Geometry: final body of the model. Coordinates: model frame, mm. A direction names the side the tool comes from. Round coordinates to 2 decimals unless told otherwise and drop trailing zeros. Order: outer loops, then holes, each group sorted by start corner. A loop starts at its lowest first (then second) coordinate and runs counter-clockwise, first axis right, second up. Notation, with made-up numbers: (69.5, -1.5) -> (115.5, -1.5) arc R13 ccw to (115.5, 7.5) -> close; hole circle Ø1 at (13, 31.5). An arc over 180 degrees is marked (long way). Put each result on its own line as item: value.
```python
from build123d import *

# Parameters (mm, degrees)
F1_DEPTH = 15.875
F3_DEPTH = 25.4
F5_DEPTH = 25.4


with BuildPart() as f1:
    # F0 (on Front) → F1 (new body)
    with BuildSketch(Plane.XZ):
        Polygon((-45.72, 0), (0, 0), (0, 12.7), (-36.195, 12.7), (-36.195, 63.5), (-45.72, 63.5), align=None)
    extrude(amount=F1_DEPTH)

    # F2 (on face) → F3 (cut)
    with BuildSketch(Plane.XY.offset(12.7)):
        with BuildLine():
            Line((-10.795, -5.3975), (-31.115, -5.3975))
            ThreePointArc((-31.115, -5.3975), (-33.655, -7.9375), (-31.115, -10.4775))
            Line((-31.115, -10.4775), (-10.795, -10.4775))
            ThreePointArc((-10.795, -10.4775), (-8.255, -7.9375), (-10.795, -5.3975))
        make_face()
    extrude(amount=-F3_DEPTH, mode=Mode.SUBTRACT)

    # F4 (on face) → F5 (cut)
    with BuildSketch(Plane(origin=(0, 0, 0), x_dir=(-1, 0, 0), z_dir=(0, 1, 0))):
        with BuildLine():
            ThreePointArc((24.13, 12.7), (25.4, 11.43), (26.67, 12.7))
            Line((26.67, 12.7), (24.13, 12.7))
        make_face()
        with BuildLine():
            Line((30.48, 12.7), (27.94, 12.7))
            ThreePointArc((27.94, 12.7), (29.21, 11.43), (30.48, 12.7))
        make_face()
        with BuildLine():
            ThreePointArc((20.32, 12.7), (21.59, 11.43), (22.86, 12.7))
            Line((22.86, 12.7), (20.32, 12.7))
        make_face()
        with BuildLine():
            Line((34.29, 12.7), (31.75, 12.7))
            ThreePointArc((31.75, 12.7), (33.02, 11.43), (34.29, 12.7))
        make_face()
        with BuildLine():
            ThreePointArc((16.51, 12.7), (17.78, 11.43), (19.05, 12.7))
            Line((19.05, 12.7), (16.51, 12.7))
        make_face()
        with BuildLine():
            ThreePointArc((12.7, 12.7), (13.97, 11.43), (15.24, 12.7))
            Line((15.24, 12.7), (12.7, 12.7))
        make_face()
        with BuildLine():
            ThreePointArc((8.89, 12.7), (10.16, 11.43), (11.43, 12.7))
            Line((11.43, 12.7), (8.89, 12.7))
        make_face()
        with BuildLine():
            ThreePointArc((5.08, 12.7), (6.35, 11.43), (7.62, 12.7))
            Line((7.62, 12.7), (5.08, 12.7))
        make_face()
        with BuildLine():
            Line((3.81, 12.7), (1.27, 12.7))
            ThreePointArc((1.27, 12.7), (2.54, 11.43), (3.81, 12.7))
        make_face()
        with BuildLine():
            ThreePointArc((3.81, 12.7), (2.54, 13.97), (1.27, 12.7))
            Line((1.27, 12.7), (3.81, 12.7))
        make_face()
    extrude(amount=-F5_DEPTH, mode=Mode.SUBTRACT)


solid = f1.part
```
1. Cut plane D-D on x = -6.35. Return loops of the section in (y, z) (3 decimals), and give its area (3 significant figures).
Ans:
outline: (-15.875, 0) -> (0, 0) -> (0, 11.43) -> (-15.875, 11.43) -> close
area: 181 mm²
2. Cut plane B-B on y = -12.75. Return loops of the section in (x, z) (3 decimals), and give its area (3 significant figures).
Ans:
outline: (-45.72, 0) -> (0, 0) -> (0, 12.7) -> (-1.27, 12.7) arc R1.27 cw to (-3.81, 12.7) -> (-5.08, 12.7) arc R1.27 cw to (-7.62, 12.7) -> (-8.89, 12.7) arc R1.27 cw to (-11.43, 12.7) -> (-12.7, 12.7) arc R1.27 cw to (-15.24, 12.7) -> (-16.51, 12.7) arc R1.27 cw to (-19.05, 12.7) -> (-20.32, 12.7) arc R1.27 cw to (-22.86, 12.7) -> (-24.13, 12.7) arc R1.27 cw to (-26.67, 12.7) -> (-27.94, 12.7) arc R1.27 cw to (-30.48, 12.7) -> (-31.75, 12.7) arc R1.27 cw to (-34.29, 12.7) -> (-36.195, 12.7) -> (-36.195, 63.5) -> (-45.72, 63.5) -> close
area: 1,040 mm²
3. Set-up query: faces 1 (the face through (-23, -11, 0)), 2 (the face through (-33.654, -7.882, 6.439)), 3 (the face through (-35, -8, 12.7)). Return all of +Z, -Z, +X, -X, +Y, -Y with unobstructed straight access to the full face (end or side cutting, diameter ignored); none if empty.
Ans:
face 1: -Z, +X, -X, +Y, -Y
face 2: +Z, -Z
face 3: +Z, +X, +Y, -Y
4. Material intervals for probe 1 along X at (y, z) = (-15, 14.5) (3 decimals); probe 2 along Z at (x, y) = (-10, -12.25); probe 3 along Z at (x, y) = (-4, -2), sorted ascending.
Ans:
probe 1: -45.72 to -36.195
probe 2: 0 to 11.44
probe 3: 0 to 12.7
5. Cut plane C-C on z = 39.5. Return loops of the section in (x, y) (3 decimals), and give its area (3 significant figures).
Ans:
outline: (-45.72, -15.875) -> (-36.195, -15.875) -> (-36.195, 0) -> (-45.72, 0) -> close
area: 151 mm²
6. Contact query for flat-ended pins moving along their axis: P1, Ø1, axis at x = -12, y = -13.5, coming from the +Z side; P2, Ø1, axis at y = -12, z = 55.5, coming from the +X side (3 decimals). Output: stop coordinate, or through.
Ans:
P1: z = 12.7
P2: x = -36.195
7. Draft query along X for faces 4 (the face through (-38, 0, 18)), 5 (the face through (-13.94, -13.14, 11.43)), 6 (the face through (0, -8, 6)). Return one class per face: +X half, -X half, draft (parallel to the pull), parting line (faces both ways), or undercut.
Ans:
face 4: draft
face 5: undercut
face 6: +X half
8. Cut plane A-A on x = -29.21. Return loops of the section in (y, z) (1 decimal).
Ans:
outline: (-15.9, 0) -> (-10.5, 0) -> (-10.5, 11.4) -> (-15.9, 11.4) -> close; (-5.4, 0) -> (0, 0) -> (0, 11.4) -> (-5.4, 11.4) -> close
